Part model, mm, in its own coordinate system. A direction names the side the tool comes from. Coordinates: 2 decimals unless noted, no trailing zeros. Loops run counter-clockwise (first coordinate to the right, second up) from the corner with the lowest first, then second, coordinate; pieces in that order, holes last. Notation, with made-up numbers: M -12.75,65 L 26.25,65 A12 ccw 26.25,84 Z; hole C 5,2 d4. An arc over 180 degrees is marked long. Use a Markdown table: item, result. Add a question column.
1) Wall check: probe 1 along Y at (x, z) = (-3.4, 2.5); probe 2 along Y at (x, z) = (-3.4, 0.45); probe 3 along Y at (x, z) = (-105, 1.3). Give the ranges that are in metal, low to high. Write a range as from..to.
2) Band-saw the part on B-B (z = 0.8). List the corners of the cut face in (x, y).
3) Band-saw the part on D-D (x = -105). List the corners of the cut face in (y, z).
4) Tool access for faces 1 (the flat face through (0, 34, 1)), 2 (the flat face through (-154, 65, 2)), 3 (the flat face through (-128, 20, 2)): list every direction of +Z, -Z, +X, -X, +Y, -Y with a clear straight run to the whole face (end or side of a thin tool).
5) Pin check, flat tips, straight feed: pin 1 Ø1.8 at (x, y) = (-150, 65.5) entering from +Z; pin 2 Ø2.5 at (x, y) = (-3.4, 64.6) entering from +Z. Stop position of each tip, or through.
6) Pull direction Y, two halves, no side cores. Call faces 4 (the flat face through (-128, 33.8, 2)), 5 (the flat face through (-79, 68, 1)), 6 (the flat face through (-79, 0, 1)), 7 (the flat face through (-155, 34, 1)): released by +Y, released by -Y, zero draft, split by the parting line, or undercut.
7) Band-saw the part on C-C (y = 64.6). List the corners of the cut face in (x, z).
8) Band-saw the part on A-A (x = -3.4). List the corners of the cut face in (y, z), plus the area to 3 significant figures.
from build123d import *

# Parameters (mm, degrees)
IZIM1_W                     = 155
IZIM1_H                     = 68
Y_KSEKLIK_EKSTR_ZYON1_DEPTH = 3
IZIM2_R                     = 5.5
IZIM2_W                     = 10
IZIM2_H                     = 13.8
KES_EKSTR_ZYON1_DEPTH       = 3
IZIM3_R                     = 2
KES_EKSTR_ZYON2_DEPTH       = 3
IZIM4_R                     = 3
KES_EKSTR_ZYON3_DEPTH       = 1


with BuildPart() as part:
    # Çizim1 → Yükseklik-Ekstrüzyon1 (new body)
    with BuildSketch(Plane.XY):
        with Locations((-77.5, 34)):
            Rectangle(IZIM1_W, IZIM1_H)
    extrude(amount=Y_KSEKLIK_EKSTR_ZYON1_DEPTH)

    # Çizim2 → Kes-Ekstrüzyon1 (cut)
    with BuildSketch(Plane.XY.offset(3)):
        with Locations((-105, 25)):
            Circle(IZIM2_R)
        with Locations((-128, 26.9)):
            Rectangle(IZIM2_W, IZIM2_H)
    extrude(amount=-KES_EKSTR_ZYON1_DEPTH, mode=Mode.SUBTRACT)

    # Çizim3 → Kes-Ekstrüzyon2 (cut)
    with BuildSketch(Plane.XY.offset(3)):
        with Locations((-151.6, 64.6)):
            Circle(IZIM3_R)
        with Locations(Location((-3.4, 64.6, 0), (0, 0, 180))):
            Circle(IZIM3_R)
        with Locations(Location((-151.6, 3.4, 0), (0, 0, 180))):
            Circle(IZIM3_R)
        with Locations((-3.4, 3.4)):
            Circle(IZIM3_R)
    extrude(amount=-KES_EKSTR_ZYON2_DEPTH, mode=Mode.SUBTRACT)

    # Çizim4 → Kes-Ekstrüzyon3 (cut)
    with BuildSketch(Plane.XY.offset(3)):
        with Locations((-151.6, 64.6)):
            Circle(IZIM4_R)
        with Locations(Location((-3.4, 64.6, 0), (0, 0, 180))):
            Circle(IZIM4_R)
        with Locations((-3.4, 3.4)):
            Circle(IZIM4_R)
        with Locations(Location((-151.6, 3.4, 0), (0, 0, 180))):
            Circle(IZIM4_R)
    extrude(amount=-KES_EKSTR_ZYON3_DEPTH, mode=Mode.SUBTRACT)


solid = part.part
Entries:
| question | item | result |
|---|---|---|
| 1 | probe 1 | 0..0.4, 6.4..61.6, 67.6..68 |
| 1 | probe 2 | 0..1.4, 5.4..62.6, 66.6..68 |
| 1 | probe 3 | 0..19.5, 30.5..68 |
| 2 | outline | M -155,0 L 0,0 L 0,68 L -155,68 Z; hole C -151.6,3.4 d4; hole C -151.6,64.6 d4; hole M -133,20 L -123,20 L -123,33.8 L -133,33.8 Z; hole C -105,25 d11; hole C -3.4,3.4 d4; hole C -3.4,64.6 d4 |
| 3 | outline | M 0,0 L 19.5,0 L 19.5,3 L 0,3 Z; M 30.5,0 L 68,0 L 68,3 L 30.5,3 Z |
| 4 | face 1 | +Z, -Z, +X, +Y, -Y |
| 4 | face 2 | +Z |
| 4 | face 3 | +Z, -Z |
| 5 | pin 1 | z = 2 |
| 5 | pin 2 | through |
| 6 | face 4 | undercut |
| 6 | face 5 | released by +Y |
| 6 | face 6 | released by -Y |
| 6 | face 7 | zero draft |
| 7 | outline | M -155,0 L -153.6,0 L -153.6,2 L -154.6,2 L -154.6,3 L -155,3 Z; M -149.6,0 L -5.4,0 L -5.4,2 L -6.4,2 L -6.4,3 L -148.6,3 L -148.6,2 L -149.6,2 Z; M -1.4,0 L 0,0 L 0,3 L -0.4,3 L -0.4,2 L -1.4,2 Z |
| 8 | outline | M 0,0 L 1.4,0 L 1.4,2 L 0.4,2 L 0.4,3 L 0,3 Z; M 5.4,0 L 62.6,0 L 62.6,2 L 61.6,2 L 61.6,3 L 6.4,3 L 6.4,2 L 5.4,2 Z; M 66.6,0 L 68,0 L 68,3 L 67.6,3 L 67.6,2 L 66.6,2 Z |
| 8 | area | 176 mm2 |
